from build123d import *

# Parameters (mm, degrees)
SKETCH2_R               = 5.75
BOSS_EXTRUDE1_DEPTH     = 7.5
CUT_EXTRUDE1_DEPTH      = 2
CUT_EXTRUDE1_DEPTH_BACK = 13.879246872
SKETCH3_R               = 1.5
SKETCH4_R               = 62.5
BOSS_EXTRUDE2_DEPTH     = 5
SKETCH5_R               = 52.5
BOSS_EXTRUDE3_DEPTH     = 10
SKETCH6_R               = 62.5
BOSS_EXTRUDE4_DEPTH     = 5
FILLET2_R               = 5


with BuildPart() as part:
    # Sketch2 → Boss-Extrude1 (new body)
    with BuildSketch(Plane.XY):
        Circle(SKETCH2_R)
        with BuildLine():
            Line((-1.25, -3), (1.25, -3))
            ThreePointArc((1.25, -3), (0, 3.25), (-1.25, -3))
        make_face(mode=Mode.SUBTRACT)
    extrude(amount=BOSS_EXTRUDE1_DEPTH)

    # Sketch3 → Cut-Extrude1 (cut, two sides: drawn at the far end of the back side and taken through both)
    with BuildSketch(Plane(origin=(0, -3, 0), x_dir=(1, 0, 0), z_dir=(0, 1, 0)).offset(-CUT_EXTRUDE1_DEPTH_BACK)):
        with Locations(Location((0, -3.75, 0), (0, 0, 90))):
            Circle(SKETCH3_R)
    extrude(amount=CUT_EXTRUDE1_DEPTH + CUT_EXTRUDE1_DEPTH_BACK, mode=Mode.SUBTRACT)

    # Sketch4 → Boss-Extrude2 (add)
    with BuildSketch(Plane.XY.offset(7.5)):
        Circle(SKETCH4_R)
    extrude(amount=BOSS_EXTRUDE2_DEPTH)

    # Sketch5 → Boss-Extrude3 (add)
    with BuildSketch(Plane.XY.offset(12.5)):
        Circle(SKETCH5_R)
    extrude(amount=BOSS_EXTRUDE3_DEPTH)

    # Sketch6 → Boss-Extrude4 (add)
    with BuildSketch(Plane.XY.offset(22.5)):
        Circle(SKETCH6_R)
    extrude(amount=BOSS_EXTRUDE4_DEPTH)

    # Fillet2
    fillet2_edges = [part.edges().sort_by_distance(p)[0] for p in [
        (-52.5, 0, 12.5),
        (-52.5, 0, 22.5),
    ]]
    fillet(fillet2_edges, radius=FILLET2_R - 0.0001)  # a hair under: the kernel refuses the full size


solid = part.part
Verification items for the finished model (mm, model axes). A direction names the side the tool comes from. Give positions to 0.01 mm unless a question says otherwise; leave off trailing zeros. Order: outer loops, then holes, each group sorted by start corner. A loop starts at its lowest first (then second) coordinate and runs counter-clockwise, first axis right, second up. Notation, with made-up numbers: M 50.5,44 L 109.5,44 A27 cw 109.5,73 Z; hole C -19.5,72.25 d11. An arc over 180 degrees is marked long. Answer as a JSON object with one key per item and string values. Group by question number.
1) Scan lines: line 1 along Z through (x, y) = (21, -53); line 2 along Z through (x, y) = (-16.5, -30); line 3 along X through (y, z) = (0.5, 6). Record each from-to range of solid material in increasing order. Write a range as [from, to].
2) Cross-section at C-C (z = 20.75). Enter the section's corners in (x, y).
3) Depth check by flat-ended pin: pin 1 Ø10 at (y, z) = (36, 3.5) entering from +X; pin 2 Ø3 at (y, z) = (-11.5, 22.5) entering from +X; pin 3 Ø4 at (x, y) = (0, 0) entering from -Z. Enter the tip coordinate at first touch or a pass-through.
4) Mould release check, pull along Z, two halves, no side actions. Record for faces 5 (the face through (-62.44, 2.75, 9.96)), 6 (the face through (27, -51, 22.5)), 7 (the face through (-1, -13, 7.5)): released by +Z, released by -Z, zero draft, split by the parting line, or undercut.
5) Cross-section at B-B (z = 9.25). Enter the section's corners in (x, y).
6) Access from +Z, -Z, +X, -X, +Y, -Y to the whole of each face (thin tool, end or side, straight path). Record for faces 1 (the face through (-62.44, 2.75, 24.96)), 2 (the face through (-0.07, -4.34, 5.25)), 3 (the face through (27, -51, 12.5)), 4 (the face through (0.125, 3.248, 3.698)).
Result sheet:
{
 "1": {"line 1": "z = [7.5, 12.52], [22.48, 27.5]", "line 2": "z = [7.5, 27.5]", "line 3": "x = [-5.73, -3.21], [3.21, 5.73]"},
 "2": {"outline": "C 0,0 d107.4"},
 "3": {"pin 1": "stops at x = 53.08", "pin 2": "stops at x = 61.69", "pin 3": "stops at z = 7.5"},
 "4": {"face 5": "zero draft", "face 6": "undercut", "face 7": "released by -Z"},
 "5": {"outline": "C 0,0 d125"},
 "6": {"face 1": "+Z, -Z", "face 2": "-Y", "face 3": "none", "face 4": "-Z"}
}
